CAD build for the part. Positions are in the model's coordinates, mm. Face numbers are marked on the shaded views. Give positions to 0.01 mm unless a question says otherwise; leave off trailing zeros. Loops run counter-clockwise (first coordinate to the right, second up) from the corner with the lowest first, then second, coordinate; pieces in that order, holes last. Notation, with made-up numbers: (-7, 40) - (7, 40) arc R14 ccw to (7, 60) - close; hole circle Ø5 at (-27.5, 73). An arc over 180 degrees is marked (long way). Return JSON: item names as keys, results as strings.
from build123d import *

# Parameters (mm, degrees)
SKETCH1_W           = 63.5
SKETCH1_H           = 12.7
SKETCH1_R           = 2.667
BOSS_EXTRUDE1_DEPTH = 3.175
CHAMFER1_SIZE       = 3.175


with BuildPart() as part:
    # Sketch1 → Boss-Extrude1 (new body)
    with BuildSketch(Plane(origin=(0, 0, 0), x_dir=(1, 0, 0), z_dir=(0, 1, 0))):
        with Locations((31.75, 6.35)):
            Rectangle(SKETCH1_W, SKETCH1_H)
        with Locations(Location((19.05, 6.35, 0), (0, 0, 270))):
            Circle(SKETCH1_R, mode=Mode.SUBTRACT)
        with Locations(Location((6.35, 6.35, 0), (0, 0, 270))):
            Circle(SKETCH1_R, mode=Mode.SUBTRACT)
        with Locations(Location((57.15, 6.35, 0), (0, 0, 270))):
            Circle(SKETCH1_R, mode=Mode.SUBTRACT)
        with Locations(Location((44.45, 6.35, 0), (0, 0, 270))):
            Circle(SKETCH1_R, mode=Mode.SUBTRACT)
        with Locations(Location((31.75, 6.35, 0), (0, 0, 270))):
            Circle(SKETCH1_R, mode=Mode.SUBTRACT)
    extrude(amount=BOSS_EXTRUDE1_DEPTH)

    # Chamfer1
    chamfer1_edges = [part.edges().sort_by_distance(p)[0] for p in [
        (0, 1.5875, 0),
        (0, 1.5875, -12.7),
        (63.5, 1.5875, -12.7),
        (63.5, 1.5875, 0),
    ]]
    chamfer(chamfer1_edges, length=CHAMFER1_SIZE)


solid = part.part
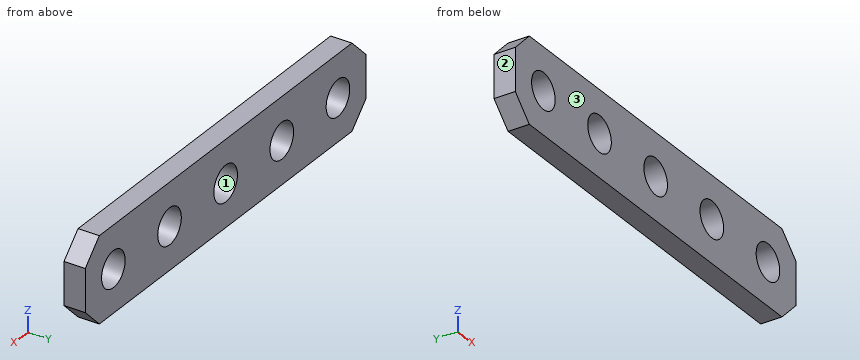
1. Cut at A-A, the plane x = 44.45. Write the cut outline in (y, z) (3 decimals).
Values follow:
{"outline": "(0, -12.7) - (3.175, -12.7) - (3.175, -9.017) - (0, -9.017) - close; (0, -3.683) - (3.175, -3.683) - (3.175, 0) - (0, 0) - close"}
2. Drill centre lines: probe 1 along X at (y, z) = (2, -6.35); probe 2 along X at (y, z) = (0.3, -7.25); probe 3 along Z at (x, y) = (32.5, 2.55). Where is each one in solid material? Low to high.
Values follow:
{"probe 1": "x = 0 to 3.68, 9.02 to 16.38, 21.72 to 29.08, 34.42 to 41.78, 47.12 to 54.48, 59.82 to 63.5", "probe 2": "x = 0 to 3.84, 8.86 to 16.54, 21.56 to 29.24, 34.26 to 41.94, 46.96 to 54.64, 59.66 to 63.5", "probe 3": "z = -12.7 to -8.91, -3.79 to 0"}
3. Pull direction X, two halves, no side cores. Call the marked faces 1, 2 and 3: +X half, -X half, draft (parallel to the pull), parting line (faces both ways), or undercut.
Values follow:
{"face 1": "undercut", "face 2": "-X half", "face 3": "draft"}
4. Cut at C-C, the plane z = -6.35. Write the cut outline in (x, y) (3 decimals), plus the area to 3 significant figures.
Values follow:
{"outline": "(0, 0) - (3.683, 0) - (3.683, 3.175) - (0, 3.175) - close; (9.017, 0) - (16.383, 0) - (16.383, 3.175) - (9.017, 3.175) - close; (21.717, 0) - (29.083, 0) - (29.083, 3.175) - (21.717, 3.175) - close; (34.417, 0) - (41.783, 0) - (41.783, 3.175) - (34.417, 3.175) - close; (47.117, 0) - (54.483, 0) - (54.483, 3.175) - (47.117, 3.175) - close; (59.817, 0) - (63.5, 0) - (63.5, 3.175) - (59.817, 3.175) - close", "area": "117 mm²"}
5. Cut at D-D, the plane x = 55.5. Write the cut outline in (y, z) (3 decimals), plus the area to 3 significant figures.
Values follow:
{"outline": "(0, -12.7) - (3.175, -12.7) - (3.175, -8.445) - (0, -8.445) - close; (0, -4.255) - (3.175, -4.255) - (3.175, 0) - (0, 0) - close", "area": "27.0 mm²"}
6. Cut at B-B, the plane y = 1.5. Write the cut outline in (x, z) (3 decimals).
Values follow:
{"outline": "(0, -9.525) - (3.175, -12.7) - (60.325, -12.7) - (63.5, -9.525) - (63.5, -3.175) - (60.325, 0) - (3.175, 0) - (0, -3.175) - close; hole circle Ø5.334 at (6.35, -6.35); hole circle Ø5.334 at (19.05, -6.35); hole circle Ø5.334 at (31.75, -6.35); hole circle Ø5.334 at (44.45, -6.35); hole circle Ø5.334 at (57.15, -6.35)"}
7. Drop a flat-ended pin along its axis: P1, Ø3, axis at x = 44.45, z = -6.35, coming from the -Y side. Give the stop position or say it passes through.
Values follow:
{"P1": "passes through"}
